The listing builds one solid part. Answer for the finished solid, in the listing's coordinates (mm). Round coordinates to 2 decimals unless told otherwise and drop trailing zeros. Write each loop counter-clockwise with the first axis right and the second up, starting at its lowest first coordinate (ties: lowest second). Pieces come first, ordered by that corner, then holes.
(1) A cutting plane is placed at B-B, the plane z = 26. Give the vertices of the cut face in (x, y), and give its area (3 significant figures).
(2) The mould has two halves that part along X. Classify faces 1 (the face through (2.26, 4.2, 19.07)), 2 (the face through (0, 6, 76)), 3 (the face through (4.2, 5.77, 147.77)): +X half, -X half, draft (parallel to the pull), parting line (faces both ways), or undercut.
(3) A cutting plane is placed at C-C, the plane y = 5.7. Give the number of separate pieces and of enclosed holes in the cut face, and give its area (3 significant figures).
(4) A cutting plane is placed at A-A, the plane x = 10. Give the vertices of the cut face in (y, z), and give its area (3 significant figures).
(5) Find the intervals of material crossed by probe 1 along Z at (x, y) = (8.85, 5.7); probe 2 along Y at (x, z) = (5.5, 81); probe 3 along Z at (x, y) = (9.25, 4.75), in increasing order.
from build123d import *

# Parameters (mm, degrees)
SKETCH_W     = 11.4
SKETCH_H     = 11.4
SKETCH_R     = 1.5
PAD_DEPTH    = 153.35
SKETCH001_R  = 1.5
POCKET_DEPTH = 11.401


with BuildPart() as part:
    # Sketch → Pad (new body)
    with BuildSketch(Plane.XY):
        with Locations((5.7, 5.7)):
            Rectangle(SKETCH_W, SKETCH_H)
        with Locations((5.7, 5.7)):
            Circle(SKETCH_R, mode=Mode.SUBTRACT)
    extrude(amount=PAD_DEPTH)

    # Sketch001 → Pocket (cut, through all)
    with BuildSketch(Plane.YZ.offset(11.4)):
        with Locations((5.7, 142.35)):
            Circle(SKETCH001_R)
        with Locations((5.7, 134.35)):
            Circle(SKETCH001_R)
        with Locations((5.7, 19)):
            Circle(SKETCH001_R)
        with Locations((5.7, 11)):
            Circle(SKETCH001_R)
    extrude(amount=-POCKET_DEPTH, mode=Mode.SUBTRACT)


solid = part.part
Solutions:
1. outline: (0, 0) - (11.4, 0) - (11.4, 11.4) - (0, 11.4) - close; hole circle Ø3 at (5.7, 5.7)
1. area: 123 mm2
2. face 1: draft
2. face 2: -X half
2. face 3: undercut
3. separate pieces: 10
3. enclosed holes: 0
3. area: 1,190 mm2
4. outline: (0, 0) - (11.4, 0) - (11.4, 153.35) - (0, 153.35) - close; hole circle Ø3 at (5.7, 11); hole circle Ø3 at (5.7, 19); hole circle Ø3 at (5.7, 134.35); hole circle Ø3 at (5.7, 142.35)
4. area: 1,720 mm2
5. probe 1: z = 0 to 9.5, 12.5 to 17.5, 20.5 to 132.85, 135.85 to 140.85, 143.85 to 153.35
5. probe 2: y = 0 to 4.21, 7.19 to 11.4
5. probe 3: z = 0 to 9.84, 12.16 to 17.84, 20.16 to 133.19, 135.51 to 141.19, 143.51 to 153.35
